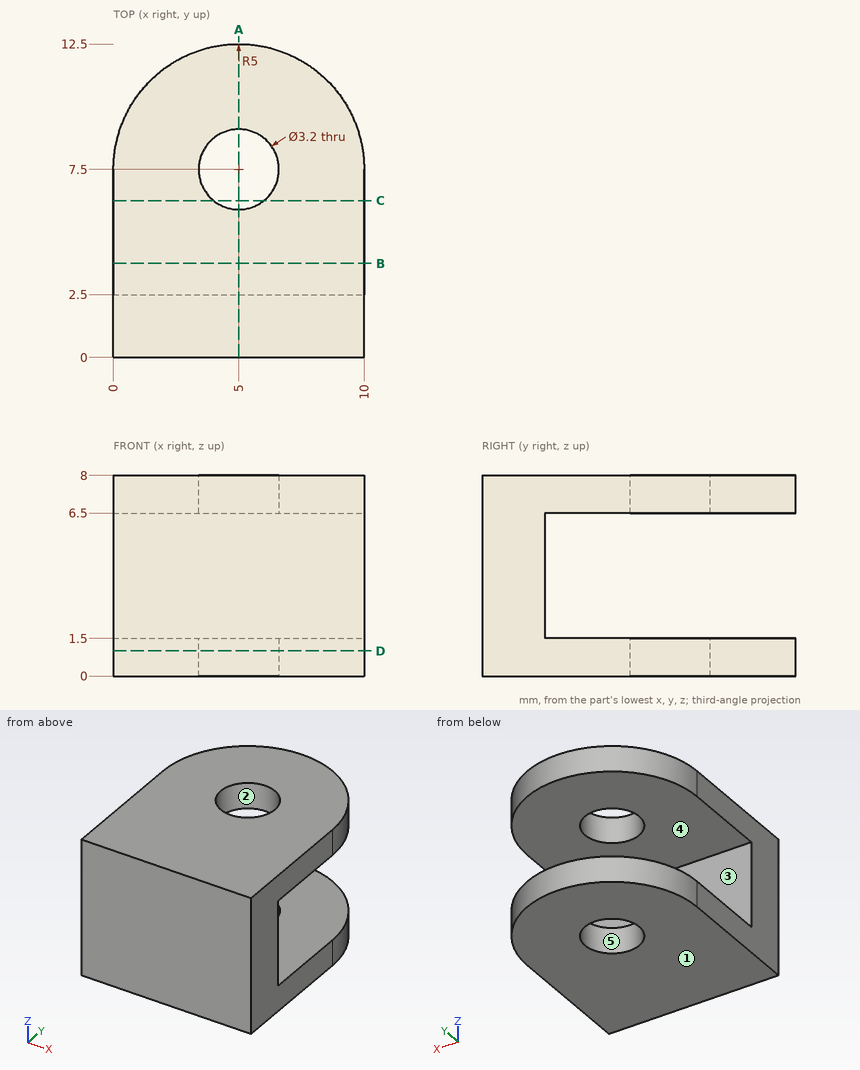
For this review, use the dimensioned drawing (mm, ordinates from the lowest corner) and the shaded views. A direction names the side the tool comes from. Coordinates: 2 decimals unless noted, no trailing zeros. Write each loop counter-clockwise with the first axis right and the second up, starting at its lowest first coordinate (ties: lowest second). Pieces come first, ordered by that corner, then holes. Notation, with made-up numbers: (-21, 60.5) -> (12, 60.5) arc R16 ccw to (12, 76.5) -> close; hole circle Ø1 at (72, 55.25). An arc over 180 degrees is marked (long way). Write each question's results on one line, items separated by ' | '. Start each with the question number.
(1) Take a section at C-C on y = 6.25. Write out the cut boundary in (x, z).
(2) Tool access review of the marked faces 4 and 5: name each direction out of +Z, -Z, +X, -X, +Y, -Y from which nothing blocks a thin tool from reaching the whole face with its end or side.
(3) Take a section at D-D on z = 1. Write out the cut boundary in (x, y).
(4) For line 1 along Y through (x, z) = (5, 7.3); line 2 along Z through (x, y) = (8, 10.5); line 3 along Y through (x, z) = (7.25, 5.75), list the stretches that pass through material, from the lowest coordinate up. Write a range as from..to.
(5) The part is to be moulded in two halves that separate along Z. For the marked faces 1, 2 and 3, say which applies: pulls with the +Z half, pulls with the -Z half, needs draft (parallel to the pull), parting line crosses it, or undercut.
(6) Take a section at B-B on y = 3.75. Write out the cut boundary in (x, z).
(7) Clearance check with flat-ended pins moving along their axes: P1, Ø2, axis at x = 8.5, z = 7, coming from the +Y side; P2, Ø4, axis at x = 3.5, z = 4, coming from the +Y side. State where each tip first meets the part, or that it passes through.
(8) Take a section at A-A on x = 5. Write out the cut boundary in (y, z).
Results found:
1) outline: (0, 0) -> (4, 0) -> (4, 1.5) -> (0, 1.5) -> close; (0, 6.5) -> (4, 6.5) -> (4, 8) -> (0, 8) -> close; (6, 0) -> (10, 0) -> (10, 1.5) -> (6, 1.5) -> close; (6, 6.5) -> (10, 6.5) -> (10, 8) -> (6, 8) -> close
2) face 4: +X, -X, +Y | face 5: +Z, -Z
3) outline: (0, 0) -> (10, 0) -> (10, 7.5) arc R5 ccw to (0, 7.5) -> close; hole circle Ø3.2 at (5, 7.5)
4) line 1: y = 0..5.9, 9.1..12.5 | line 2: z = 0..1.5, 6.5..8 | line 3: y = 0..2.5
5) face 1: pulls with the -Z half | face 2: needs draft | face 3: undercut
6) outline: (0, 0) -> (10, 0) -> (10, 1.5) -> (0, 1.5) -> close; (0, 6.5) -> (10, 6.5) -> (10, 8) -> (0, 8) -> close
7) P1: stops at y = 11.83 | P2: stops at y = 2.5
8) outline: (0, 0) -> (5.9, 0) -> (5.9, 1.5) -> (2.5, 1.5) -> (2.5, 6.5) -> (5.9, 6.5) -> (5.9, 8) -> (0, 8) -> close; (9.1, 0) -> (12.5, 0) -> (12.5, 1.5) -> (9.1, 1.5) -> close; (9.1, 6.5) -> (12.5, 6.5) -> (12.5, 8) -> (9.1, 8) -> close
